Geometry: see drawing. Coordinates: mm, zero at the bounding-box minimum. A direction names the side the tool comes from. Coordinates: 2 decimals unless noted, no trailing zeros. Write each loop counter-clockwise with the first axis right and the second up, starting at its lowest first coordinate (ties: lowest second). Pieces come first, ordered by that corner, then holes. Notation, with made-up numbers: M 76.5,-3 L 113.5,-3 A24 ccw 113.5,24 Z; hole C -32,28.25 d7. An arc over 180 degrees is marked long. Write item = value, one per line. Start each with the question number.
1. Pin query (flat end, axial travel): pin 1 Ø18 at (x, y) = (20, 20) entering from -Z; pin 2 Ø8 at (x, y) = (30.5, 25) entering from -Z; pin 3 Ø4 at (x, z) = (29.5, 3) entering from -Y; pin 4 Ø3 at (x, y) = (7.5, 35) entering from +Z. Return the tip coordinate at first contact, or that it passes through.
2. Pull-direction query (X, two-part tool) for the marked faces 1, 2 and 3; classes: pulls with the +X half, pulls with the -X half, needs draft (parallel to the pull), parting line crosses it, or undercut.
3. Line query: line 1 along X through (y, z) = (20, 2.3); line 2 along Y through (x, z) = (20, 8.1); line 3 along Y through (x, z) = (20, 1.45). Output: solid intervals per line, ascending.
4. Section query C-C (x = 35.5). Output: boundary loops of the cut face in (y, z).
5. Section query D-D (z = 4.5). Output: boundary loops of the cut face in (x, y), then the cut area to 3 significant figures.
6. Section query A-A (x = 20). Output: boundary loops of the cut face in (y, z), then the cut area to 3 significant figures.
7. Access query for the marked faces 4, 5 and 6. Directions: +Z, -Z, +X, -X, +Y, -Y. A direction counts if a zero-diameter tool reaches every point of the face in a straight line with its end or side. Return the directions, or none.
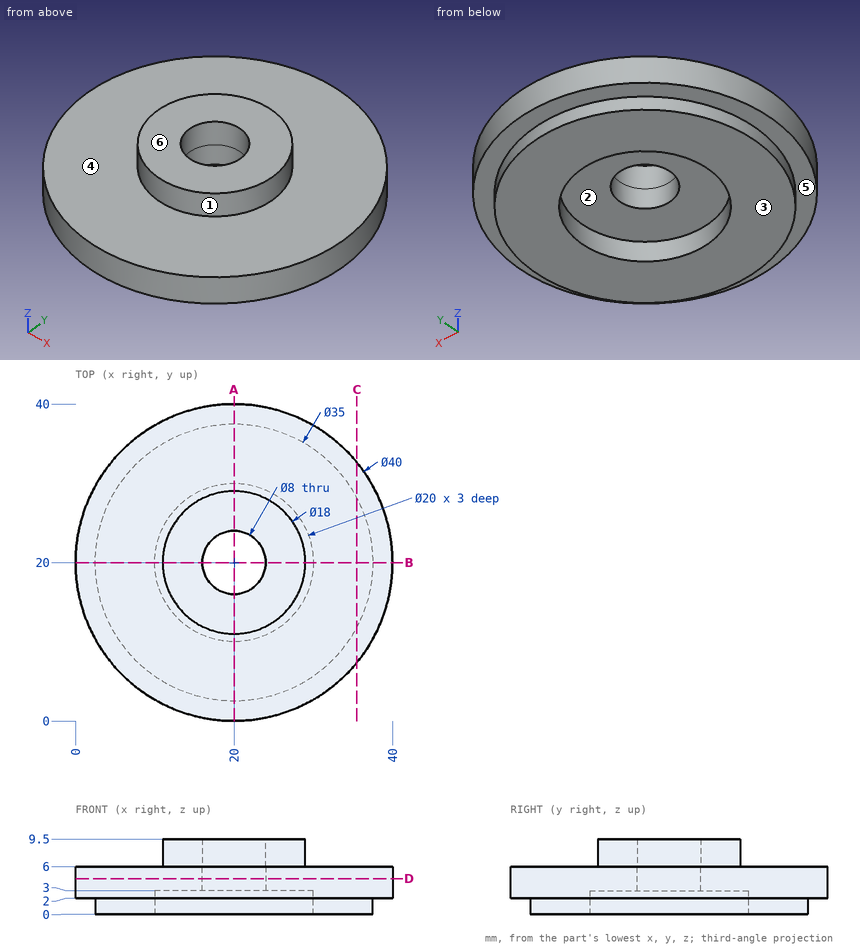
Results are:
q1.pin_1 = 3
q1.pin_2 = 0
q1.pin_3 = 1.46
q1.pin_4 = 6
q2.face_1 = parting line crosses it
q2.face_2 = undercut
q2.face_3 = needs draft
q3.line_1 = 0 to 10, 30 to 40
q3.line_2 = 11 to 16, 24 to 29
q3.line_3 = 2.5 to 10, 30 to 37.5
q4.outline = M 7.36,2 L 11.88,2 L 11.88,0 L 28.12,0 L 28.12,2 L 32.64,2 L 32.64,6 L 7.36,6 Z
q5.outline = C 20,20 d40; hole C 20,20 d8
q5.area = 1,210 mm^2
q6.outline = M 0,2 L 2.5,2 L 2.5,0 L 10,0 L 10,3 L 16,3 L 16,9.5 L 11,9.5 L 11,6 L 0,6 Z; M 24,3 L 30,3 L 30,0 L 37.5,0 L 37.5,2 L 40,2 L 40,6 L 29,6 L 29,9.5 L 24,9.5 Z
q6.area = 181 mm^2
q7.face_4 = +Z
q7.face_5 = -Z
q7.face_6 = +Z, +X, -X, +Y, -Y
